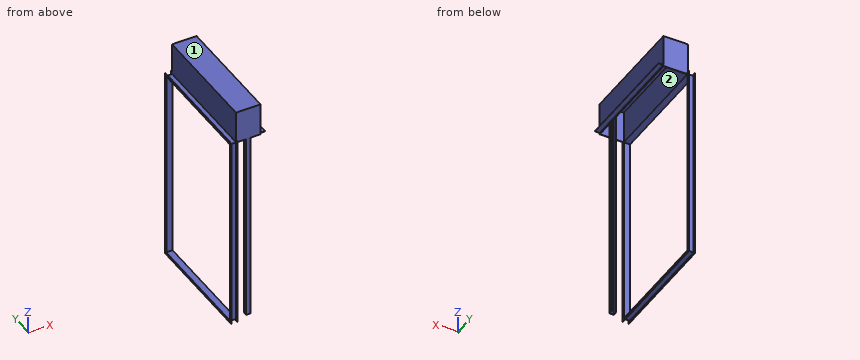
```python
from build123d import *

# Parameters (mm, degrees)
F0_W      = 30
F0_H      = 2
F1_DEPTH  = 710
F8_DEPTH  = 1414
F9_W      = 154
F9_H      = 206
F10_DEPTH = 2
F11_W     = 154
F11_H     = 206
F12_DEPTH = 2


with BuildPart() as f1:
    # F0 (on Front) → F1 (new body)
    with BuildSketch(Plane.XZ):
        Polygon((-2, 0), (0, 0), (0, 8), (0, 10), (0, 206), (-154, 206), (-154, 0), (-152, 0), (-152, 204), (-2, 204), align=None)
        with Locations((15, 9)):
            Rectangle(F0_W, F0_H)
    extrude(amount=-F1_DEPTH)

    # F6: sweep along a path in F3
    with BuildLine(Plane.YZ.offset(-152)) as f6_path:
        Line((0, 0), (710, 0))
        Line((710, 0), (710, -1210))
        Line((710, -1210), (0, -1210))
        Line((0, -1210), (0, 0))
    # F5 (on offset) → F6 (sweep)
    with BuildSketch(Plane.XZ):
        Polygon((-192, 0), (-152, 0), (-152, 15), (-154, 15), (-154, 2), (-190, 2), (-190, 15), (-192, 15), align=None)
    sweep(path=f6_path.line, transition=Transition.RIGHT)

    # F7 (on face) → F8 (join, through all)
    with BuildSketch(Plane(origin=(0, 0, 204), x_dir=(1, 0, 0), z_dir=(0, 0, -1))):
        Polygon((-75, 0), (-77, 0), (-89, 0), (-89, -26), (-87, -26), (-87, -2), (-75, -2), (-63, -2), (-63, -26), (-61, -26), (-61, 0), align=None)
    extrude(amount=F8_DEPTH)

    # F9 (on face) → F10 (join)
    with BuildSketch(Plane.XZ):
        with Locations((-77, 103)):
            Rectangle(F9_W, F9_H)
    extrude(amount=F10_DEPTH)

    # F11 (on face) → F12 (join)
    with BuildSketch(Plane(origin=(0, 710, 0), x_dir=(-1, 0, 0), z_dir=(0, 1, 0))):
        with Locations((77, 103)):
            Rectangle(F11_W, F11_H)
    extrude(amount=F12_DEPTH)


solid = f1.part
```
Geometry check sheet. Reference: the model listing, model coordinates, mm. Face numbers are marked on the shaded views. Coordinates: 2 decimals unless noted, no trailing zeros. Write each loop counter-clockwise with the first axis right and the second up, starting at its lowest first coordinate (ties: lowest second). Pieces come first, ordered by that corner, then holes. Notation, with made-up numbers: M -12,-40 L 29,-40 A18 ccw 29,-24 Z; hole C -35,21.5 d9. An arc over 180 degrees is marked long. Use one line per item in the form item = value. Start each with the question number.
1) Release check for a two-part mould opening along Y. For the marked faces 1 and 2 record: pulls with the +Y half, pulls with the -Y half, needs draft (parallel to the pull), parting line crosses it, or undercut.
2) Section check C-C on x = -115.5. Enter the section's corners in (y, z).
3) Go/stop test with flat-tipped pins: pin 1 Ø18 at (x, y) = (-166, 368.5) entering from +Z; pin 2 Ø2 at (x, z) = (-62.5, -962.5) entering from -Y; pin 3 Ø1.6 at (x, y) = (-153.5, -6) entering from +Z; pin 4 Ø12 at (x, z) = (-154.5, -380.5) entering from -Y. Record where each tip stops, or that it passes through.
4) Section check A-A on z = -412.5. Enter the section's corners in (x, y), and give its area (3 significant figures).
5) Section check B-B on y = 430. Enter the section's corners in (x, z).
6) Thickness scan on probe 1 along X at (y, z) = (454, 5.5); probe 2 along Y at (x, z) = (-178, -1147); probe 3 along Z at (x, y) = (-166, 525). Record the ranges inside material, lowest first. Write a range as from..to.
Responses:
q1.face_1 = needs draft
q1.face_2 = undercut
q2.outline = M -2,0 L 0,0 L 0,204 L 710,204 L 710,0 L 712,0 L 712,206 L -2,206 Z
q3.pin_1 = 2
q3.pin_2 = 0
q3.pin_3 = 15
q3.pin_4 = -15
q4.outline = M -192,-15 L -190,-15 L -190,-2 L -154,-2 L -154,-15 L -152,-15 L -152,0 L -192,0 Z; M -192,710 L -152,710 L -152,725 L -154,725 L -154,712 L -190,712 L -190,725 L -192,725 Z; M -89,0 L -61,0 L -61,26 L -63,26 L -63,2 L -87,2 L -87,26 L -89,26 Z
q4.area = 416 mm2
q5.outline = M -192,-1225 L -190,-1225 L -190,-1212 L -154,-1212 L -154,-1225 L -152,-1225 L -152,-1210 L -192,-1210 Z; M -192,0 L -152,0 L -152,204 L -2,204 L -2,0 L 0,0 L 0,8 L 30,8 L 30,10 L 0,10 L 0,206 L -154,206 L -154,2 L -190,2 L -190,15 L -192,15 Z
q6.probe_1 = -192..-190, -154..-152, -2..0
q6.probe_2 = -2..0, 710..712
q6.probe_3 = -1212..-1210, 0..2
